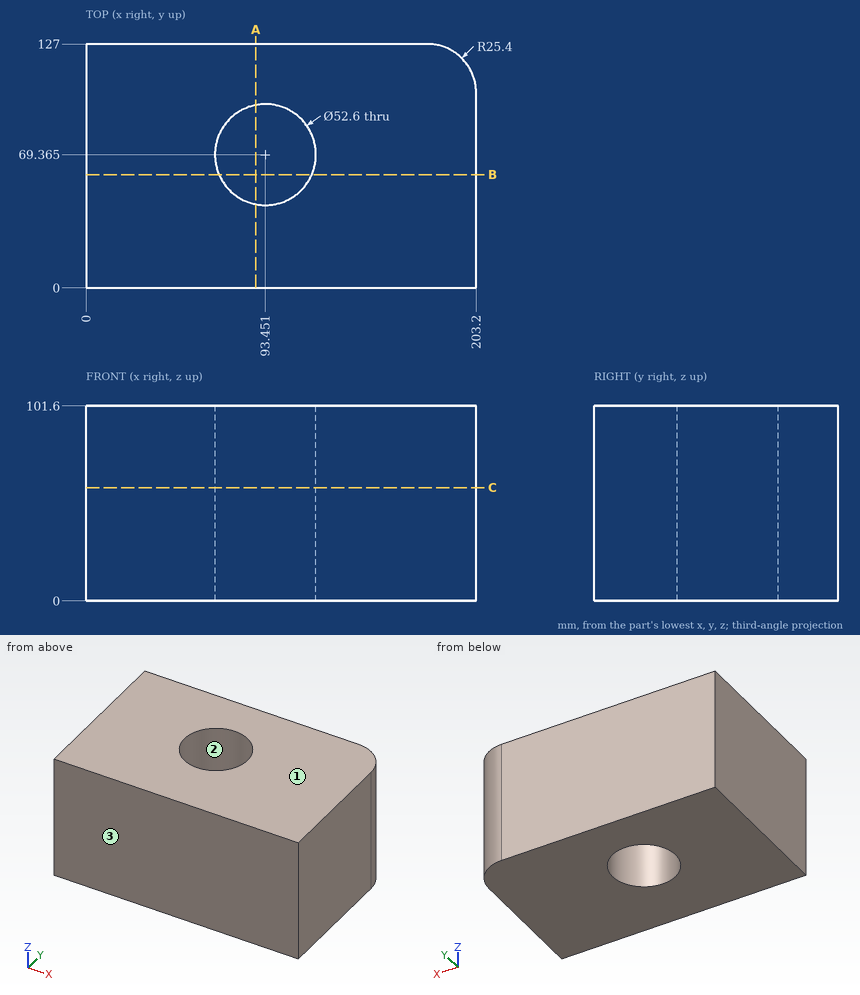
Print and shaded views of the part. All mm, measured from the part's lowest x, y and z. Coordinates: 2 decimals unless noted, no trailing zeros. Order: outer loops, then holes, each group sorted by start corner. A loop starts at its lowest first (then second) coordinate and runs counter-clockwise, first axis right, second up. Notation, with made-up numbers: (-7, -28) - (32, -28) arc R32 ccw to (32, 10) - close; hole circle Ø4 at (79.25, 20.25). An arc over 180 degrees is marked (long way). Put each result on its own line as item: value.
1. Drop a flat-ended pin along its axis: P1, Ø5, axis at y = 106, z = 70, coming from the +X side. Give the stop position or say it passes through.
Answer sheet:
P1: stops at x = 203.13
2. Saw through at C-C (z = 59). Write the cut outline in (x, y) (1 decimal).
Answer sheet:
outline: (0, 0) - (203.2, 0) - (203.2, 101.6) arc R25.4 ccw to (177.8, 127) - (0, 127) - close; hole circle Ø52.6 at (93.5, 69.4)
3. Probe line 1 along Y through (x, z) = (83.5, 54); line 2 along X through (y, z) = (92, 31) (1 decimal); line 3 along Y through (x, z) = (73, 56). List the from-to ranges inside material, lowest first. Write a range as [from, to].
Answer sheet:
line 1: y = [0, 45.02], [93.71, 127]
line 2: x = [0, 80.1], [106.8, 203.2]
line 3: y = [0, 52.83], [85.9, 127]
4. Saw through at B-B (y = 59). Write the cut outline in (x, z), and give its area (3 significant figures).
Answer sheet:
outline: (0, 0) - (69.28, 0) - (69.28, 101.6) - (0, 101.6) - close; (117.62, 0) - (203.2, 0) - (203.2, 101.6) - (117.62, 101.6) - close
area: 15,700 mm^2
5. Pull direction Y, two halves, no side cores. Call the marked faces 1, 2 and 3: pulls with the +Y half, pulls with the -Y half, needs draft (parallel to the pull), parting line crosses it, or undercut.
Answer sheet:
face 1: needs draft
face 2: undercut
face 3: pulls with the -Y half
6. Saw through at A-A (x = 88.5). Write the cut outline in (y, z) (1 decimal).
Answer sheet:
outline: (0, 0) - (43.5, 0) - (43.5, 101.6) - (0, 101.6) - close; (95.2, 0) - (127, 0) - (127, 101.6) - (95.2, 101.6) - close
